Job drawing, mm, ordinate dimensions from the low corner. One solid piece. A direction names the side the tool comes from. Give positions to 0.01 mm unless a question says otherwise; leave off trailing zeros. Write each loop counter-clockwise with the first axis right and the second up, starting at its lowest first coordinate (ties: lowest second). Pieces come first, ordered by that corner, then holes. Notation, with made-up numbers: M 24.5,-5 L 28.5,-5 A15 ccw 28.5,22 Z; hole C 66.25,68 d4. An arc over 180 degrees is marked long. Answer as CSV lines item,"result". Start each with the question number.
1) Wall check: line 1 along Y through (x, z) = (42, 1.75) (1 decimal); line 2 along Y through (x, z) = (42, 8) (1 decimal); line 3 along Z through (x, y) = (60.5, 63). Give the ranges that are in metal, low to high. Write a range as from..to.
2) Slice it at B-B, the plane x = 42. Give the cut face in (y, z) (1 decimal), plus the area to 3 significant figures.
3) Tool access for the marked faces 4 and 5: list every direction of +Z, -Z, +X, -X, +Y, -Y with a clear straight run to the whole face (end or side of a thin tool).
4) Slice it at A-A, the plane z = 5.5. Give the number of separate pieces and of enclosed holes in the cut face, plus the area to 3 significant figures.
5) Pin check, flat tips, straight feed: pin 1 Ø2 at (y, z) = (56, 14) entering from +X (1 decimal); pin 2 Ø3 at (x, z) = (25, 24) entering from -Y; pin 3 Ø1 at (y, z) = (57.5, 13.5) entering from -X; pin 4 Ø5 at (x, y) = (74.5, 42) entering from -Z. Stop position of each tip, or through.
6) Slice it at C-C, the plane y = 33. Give the cut face in (x, z) (1 decimal), plus the area to 3 significant figures.
7) Mould opens along X. For the marked faces 1, 2 and 3 say: pulls with the +X half, pulls with the -X half, needs draft (parallel to the pull), parting line crosses it, or undercut.
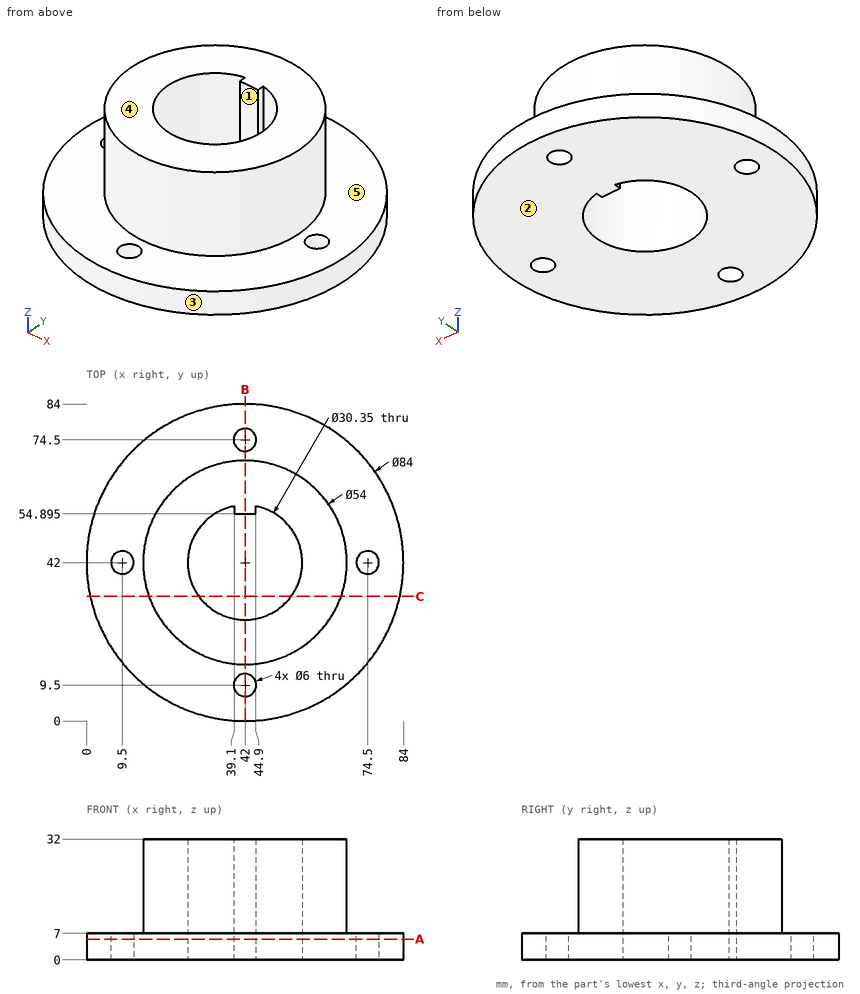
Found:
1,line 1,"0..6.5, 12.5..26.8, 54.9..71.5, 77.5..84"
1,line 2,"15..26.8, 54.9..69"
1,line 3,"0..7"
2,outline,"M 0,0 L 6.5,0 L 6.5,7 L 0,7 Z; M 12.5,0 L 26.8,0 L 26.8,32 L 15,32 L 15,7 L 12.5,7 Z; M 54.9,0 L 71.5,0 L 71.5,7 L 69,7 L 69,32 L 54.9,32 Z; M 77.5,0 L 84,0 L 84,7 L 77.5,7 Z"
2,area,"956 mm²"
3,face 4,"+Z, +X, -X, +Y, -Y"
3,face 5,"+Z"
4,separate pieces,"1"
4,enclosed holes,"5"
4,area,"4,720 mm²"
5,pin 1,"x = 65.7"
5,pin 2,"y = 19.89"
5,pin 3,"x = 19.55"
5,pin 4,"through"
6,outline,"M 1,0 L 29.8,0 L 29.8,32 L 16.5,32 L 16.5,7 L 1,7 Z; M 54.2,0 L 83,0 L 83,7 L 67.5,7 L 67.5,32 L 54.2,32 Z"
6,area,"1,070 mm²"
7,face 1,"undercut"
7,face 2,"needs draft"
7,face 3,"parting line crosses it"
